```python
from build123d import *

# Parameters (mm, degrees)
ESBO_O1_W                                      = 130
ESBO_O1_H                                      = 20
RESSALTO_EXTRUS_O1_DEPTH                       = 95
CORTE_EXTRUS_O2_REACH                          = 22
CORTE_EXTRUS_O4_DEPTH                          = 1
CORTE_EXTRUS_O4_DEPTH_BACK                     = 66
BROCA_DE_ROSQUEAR_DE_CANO_PARA_TARRAXA_D_D     = 6.579997
BROCA_DE_ROSQUEAR_DE_CANO_PARA_TARRAXA_D_DEPTH = 10
BROCA_DE_ROSQUEAR_DE_CANO_PARA_TARRAXA_D_TIP   = 1.976830535
BROCA_DE_ROSQUEAR_DE_CANO_PARA_TARRA_2_D       = 6.579997
BROCA_DE_ROSQUEAR_DE_CANO_PARA_TARRA_2_DEPTH   = 10
BROCA_DE_ROSQUEAR_DE_CANO_PARA_TARRA_2_TIP     = 1.976830535
FILETE2_R                                      = 5
ESBO_O38_W                                     = 45
ESBO_O38_H                                     = 2
CORTE_EXTRUS_O9_DEPTH                          = 40


with BuildPart() as part:
    # Esboço1 → Ressalto-extrusão1 (new body)
    with BuildSketch(Plane.XY):
        Rectangle(ESBO_O1_W, ESBO_O1_H)
    extrude(amount=RESSALTO_EXTRUS_O1_DEPTH)

    # Esboço2 → Corte-extrusão2 (cut, up to next)
    with BuildSketch(Plane(origin=(0, 10, 0), x_dir=(1, 0, 0), z_dir=(0, 1, 0)), mode=Mode.PRIVATE) as corte_extrus_o2_sk1:
        with BuildLine():
            Line((65, 0), (-20, 0))
            Line((-20, 0), (-35, -40))
            ThreePointArc((-35, -40), (-23.93419305, -71.594486486), (0, -95))
            Line((0, -95), (65, -95))
            Line((65, -95), (65, 0))
        make_face()
    corte_extrus_o2_tool1 = extrude(corte_extrus_o2_sk1.sketch, amount=-CORTE_EXTRUS_O2_REACH, mode=Mode.PRIVATE) & part.part
    add(corte_extrus_o2_tool1.solids().sort_by_distance((19.507418, 10, 46.266943))[0], mode=Mode.SUBTRACT)

    # Esboço13 → Corte-extrusão4 (cut, two sides)
    with BuildSketch(Plane.ZY.offset(65)) as corte_extrus_o4_sk:
        Polygon((-200.200134404, 50.040026881), (0, 10), (95, -9), (295.200134404, -49.040026881), (375.280188165, 351.360241926), (-120.120080642, 450.440295688), align=None)
    extrude(amount=CORTE_EXTRUS_O4_DEPTH, mode=Mode.SUBTRACT)
    extrude(corte_extrus_o4_sk.sketch, amount=-CORTE_EXTRUS_O4_DEPTH_BACK, mode=Mode.SUBTRACT)

    # Broca de rosquear de cano para tarraxa d
    with Locations(Plane.ZY.offset(65)):
        with Locations((20, -2)):
            Hole(BROCA_DE_ROSQUEAR_DE_CANO_PARA_TARRAXA_D_D / 2, depth=BROCA_DE_ROSQUEAR_DE_CANO_PARA_TARRAXA_D_DEPTH)
            with Locations((0, 0, -(BROCA_DE_ROSQUEAR_DE_CANO_PARA_TARRAXA_D_DEPTH + BROCA_DE_ROSQUEAR_DE_CANO_PARA_TARRAXA_D_TIP / 2))):  # 118° drill point
                Cone(0, BROCA_DE_ROSQUEAR_DE_CANO_PARA_TARRAXA_D_D / 2, BROCA_DE_ROSQUEAR_DE_CANO_PARA_TARRAXA_D_TIP, mode=Mode.SUBTRACT)

    # Broca de rosquear de cano para tarra 2
    with Locations(Plane(origin=(-17.534246575, 0, -6.575342466), x_dir=(0.351123442, 0, -0.936329178), z_dir=(0.936329178, 0, 0.351123442))):
        with Locations((-27.022468832, -2)):
            Hole(BROCA_DE_ROSQUEAR_DE_CANO_PARA_TARRA_2_D / 2, depth=BROCA_DE_ROSQUEAR_DE_CANO_PARA_TARRA_2_DEPTH)
            with Locations((0, 0, -(BROCA_DE_ROSQUEAR_DE_CANO_PARA_TARRA_2_DEPTH + BROCA_DE_ROSQUEAR_DE_CANO_PARA_TARRA_2_TIP / 2))):  # 118° drill point
                Cone(0, BROCA_DE_ROSQUEAR_DE_CANO_PARA_TARRA_2_D / 2, BROCA_DE_ROSQUEAR_DE_CANO_PARA_TARRA_2_TIP, mode=Mode.SUBTRACT)

    # Filete2
    filete2_edges = [part.edges().sort_by_distance(p)[0] for p in [
        (-65, -9.5, 95),
    ]]
    fillet(filete2_edges, radius=FILETE2_R)

    # Esboço38 → Corte-extrusão9 (cut)
    with BuildSketch(Plane(origin=(0, 0, 0), x_dir=(-1, 0, 0), z_dir=(0, 0, -1))):
        with Locations((42.5, -9)):
            Rectangle(ESBO_O38_W, ESBO_O38_H)
    extrude(amount=-CORTE_EXTRUS_O9_DEPTH, mode=Mode.SUBTRACT)


solid = part.part
```
For this review, take the finished solid that the model builds, in its own axes (mm). A direction names the side the tool comes from. Coordinates: 2 decimals unless noted, no trailing zeros. Write each loop counter-clockwise with the first axis right and the second up, starting at its lowest first coordinate (ties: lowest second). Pieces come first, ordered by that corner, then holes. Notation, with made-up numbers: (-0.5, 36) - (4.5, 36) arc R12 ccw to (4.5, 48) - close; hole circle Ø2 at (-16, 10.25). An arc over 180 degrees is marked (long way). Answer in a Markdown table with one row per item. Add a question column.
Q1. Tool access review of faces 5 (the flat face through (-50, -9, 40)), 6 (the cylindrical face through (-27.844, -6.583, 64.645)), 7 (the conical face through (-37.807, -1.518, 14.354)): name each direction out of +Z, -Z, +X, -X, +Y, -Y from which nothing blocks a thin tool from reaching the whole face with its end or side.
Q2. We need section C-C, the plane z = 42. State the section outline as (x, y) points.
Q3. We need section B-B, the plane y = 3.5. State the section outline as (x, z) points.
Q4. Draft analysis for pull direction Z (two halves, no side actions). For faces 1 (the cylindrical face through (-59.93, -1.012, 16.862)), 2 (the flat face through (-47, -8, 20)), 3 (the flat face through (-47.4, 0.63, 46.84)), 4 (the flat face through (-43, 1, 0)), state which applies: +Z half, -Z half, draft (parallel to the pull), parting line (faces both ways), or undercut.
Q5. For probe 1 along Y at (x, z) = (-62.5, 20); probe 2 along Y at (x, z) = (-41, 9); probe 3 along X at (y, z) = (-3.5, 6.5), list the stretches that pass through material, from the lowest coordinate up.
Q6. For P1, Ø8, axis at y = 0, z = 56, coming from the -X side; P2, Ø6, axis at y = -8, z = 21.5, coming from the +X side; P3, Ø0.6, axis at x = -44, y = -9, coming from the -Z side; P4, Ø6, axis at y = -2, z = 20, coming from the +X side, all flat-tipped, find the tip position at first contact; note any pin that passes through.
Q7. We need section A-A, the plane x = -49. State the section outline as (y, z) points.
Answer list:
| question | item | result |
|---|---|---|
| 1 | face 5 | -Z, +X, -X, -Y |
| 1 | face 6 | +X, +Y, -Y |
| 1 | face 7 | none |
| 2 | outline | (-65, -10) - (-34.76, -10) - (-34.76, 1.6) - (-65, 1.6) - close |
| 3 | outline | (-65, 0) - (-20, 0) - (-32.19, 32.5) - (-65, 32.5) - close |
| 4 | face 1 | undercut |
| 4 | face 2 | draft |
| 4 | face 3 | +Z half |
| 4 | face 4 | -Z half |
| 5 | probe 1 | y = -8 to -5.29, 1.29 to 6 |
| 5 | probe 2 | y = -8 to 8.2 |
| 5 | probe 3 | x = -65 to -22.44 |
| 6 | P1 | stops at x = -65 |
| 6 | P2 | stops at x = -26.94 |
| 6 | P3 | stops at z = 40 |
| 6 | P4 | stops at x = -27.5 |
| 7 | outline | (-10, 40) - (-8, 40) - (-8, 0) - (10, 0) - (-9, 95) - (-10, 95) - close |
